Geometry check sheet. Reference: the model listing, model coordinates, mm. A direction names the side the tool comes from. Coordinates: 2 decimals unless noted, no trailing zeros. Loops run counter-clockwise (first coordinate to the right, second up) from the corner with the lowest first, then second, coordinate; pieces in that order, holes last.
from build123d import *

# Parameters (mm, degrees)
F3_R     = 9.525
F3_R_2   = 6.980415
F4_DEPTH = 304.801


with BuildPart() as f1:
    # F0 (on Right) → F1 (revolve)
    with BuildSketch(Plane.YZ):
        Polygon((0, 76.2), (0, 114.3), (-12.7, 114.3), (-12.7, 82.55), (-292.1, 82.55), (-292.1, 114.3), (-304.8, 114.3), (-304.8, 76.2), align=None)
    revolve(axis=Axis((0, 69.986956, 0), (0, 1, 0)))

    # F3 (on offset) → F4 (cut, through all)
    with BuildSketch(Plane.XZ.offset(304.8)):
        with Locations((0, 98.425)):
            Circle(F3_R)
        with Locations((0, -98.425)):
            Circle(F3_R_2)
    extrude(amount=-F4_DEPTH, mode=Mode.SUBTRACT)


solid = f1.part
1) Material ranges on probe 1 along Y at (x, z) = (-78.5, -61); probe 2 along X at (y, z) = (-77, 0); probe 3 along Z at (x, y) = (-68, -169.5), recorded low to high.
Data:
probe 1: y = -304.8 to -292.1, -12.7 to 0
probe 2: x = -82.55 to -76.2, 76.2 to 82.55
probe 3: z = -46.8 to -34.39, 34.39 to 46.8
2) Section check B-B on z = 0. Record the cut outline in (x, y).
Data:
outline: (-114.3, -304.8) - (-76.2, -304.8) - (-76.2, 0) - (-114.3, 0) - (-114.3, -12.7) - (-82.55, -12.7) - (-82.55, -292.1) - (-114.3, -292.1) - close; (76.2, -304.8) - (114.3, -304.8) - (114.3, -292.1) - (82.55, -292.1) - (82.55, -12.7) - (114.3, -12.7) - (114.3, 0) - (76.2, 0) - close
3) Access from +Z, -Z, +X, -X, +Y, -Y to the whole of each face (thin tool, end or side, straight path). Record for faces 4 (the cylindrical face through (3.22, -298.54, -104.62)), 5 (the flat face through (-33, -292.1, -76)).
Data:
face 4: +Y, -Y
face 5: none
4) Section check D-D on x = 43.5. Record the cut outline in (y, z), and give its area (3 significant figures).
Data:
outline: (-304.8, -105.7) - (-292.1, -105.7) - (-292.1, -70.16) - (-12.7, -70.16) - (-12.7, -105.7) - (0, -105.7) - (0, -62.56) - (-304.8, -62.56) - close; (-304.8, 62.56) - (0, 62.56) - (0, 105.7) - (-12.7, 105.7) - (-12.7, 70.16) - (-292.1, 70.16) - (-292.1, 105.7) - (-304.8, 105.7) - close
area: 6,440 mm2
5) Depth check by flat-ended pin: pin 1 (15 mm diameter, centred on x = 0, z = 98.425, fed in from -Y); pin 2 (2 mm diameter, centred on x = -51, y = -43.5, fed in from -Z); pin 3 (8 mm diameter, centred on x = -68.5, y = -213.5, fed in from -Z); pin 4 (3 mm diameter, centred on y = -138.5, z = -41.5, fed in from -X). Enter the tip coordinate at first touch or a pass-through.
Data:
pin 1: passes through
pin 2: stops at z = -65.68
pin 3: stops at z = -51.52
pin 4: stops at x = -72.21
6) Section check C-C on y = -285.5. Record the cut outline in (x, z).
Data:
outline: circle Ø165.1 at (0, 0); hole circle Ø152.4 at (0, 0)
7) Mould release check, pull along Y, two halves, no side actions. Record for faces 1 (the flat face through (-24, 0, -75)), 2 (the cylindrical face through (-7.02, -298.54, 104.86)), 3 (the cylindrical face through (-80.587, -154.356, -17.895)): +Y half, -Y half, draft (parallel to the pull), parting line (faces both ways), or undercut.
Data:
face 1: +Y half
face 2: draft
face 3: undercut
8) Section check A-A on x = 0. Count the separate pieces of the cut face and the enclosed holes in it, and give its area (3 significant figures).
Data:
separate pieces: 6
enclosed holes: 0
area: 4,650 mm2
